from build123d import *

# Parameters (mm, degrees)
F0_W     = 132.985286
F0_H     = 132.985286
F1_DEPTH = 25.4


with BuildPart() as f1:
    # F0 (on Top) → F1 (new body)
    with BuildSketch(Plane.XY):
        Polygon((84.181237, -55.154049), (84.181237, 6.35), (-139.335286, 6.35), (-139.335286, -217.166522), (-77.831237, -217.166522), (-77.831237, -278.670572), (145.685286, -278.670572), (145.685286, -55.154049), align=None)
        Polygon((0, -272.320572), (-71.481237, -272.320572), (-71.481237, -210.816522), (-132.985286, -210.816522), (-132.985286, -139.335286), (0, -139.335286), align=None, mode=Mode.SUBTRACT)
        with Locations((72.842643, -205.827929)):
            Rectangle(F0_W, F0_H, mode=Mode.SUBTRACT)
        with Locations((-66.492643, -66.492643)):
            Rectangle(F0_W, F0_H, mode=Mode.SUBTRACT)
        Polygon((6.35, -132.985286), (6.35, 0), (77.831237, 0), (77.831237, -61.504049), (139.335286, -61.504049), (139.335286, -132.985286), align=None, mode=Mode.SUBTRACT)
    extrude(amount=F1_DEPTH)


solid = f1.part
Could you check a few things on this model? Use its own coordinates, in mm. A direction names the side the tool comes from. Round coordinates to 2 decimals unless told otherwise and drop trailing zeros. Write each loop counter-clockwise with the first axis right and the second up, starting at its lowest first coordinate (ties: lowest second). Pieces come first, ordered by that corner, then holes. Notation, with made-up numbers: (73.5, 88) -> (105.5, 88) arc R31 ccw to (105.5, 113) -> close; hole circle Ø11 at (-24, 66). An arc over 180 degrees is marked (long way). Use a Markdown table: item, result.
1. We'd pull the mould along Y, two halves only. Please class faces 1 (the face through (115, -55.154, 13)), 2 (the face through (-132.985, -67, 13)), 3 (the face through (3, -135, 25.4)): +Y half, -Y half, draft (parallel to the pull), parting line (faces both ways), or undercut.
Answer key:
| item | result |
|---|---|
| face 1 | +Y half |
| face 2 | undercut |
| face 3 | draft |
2. For pin 1 Ø7.5 at (x, z) = (-122, 14) entering from -Y; pin 2 Ø7.5 at (x, z) = (93, 10.5) entering from +Y, each with a flat end and sliding along its axis, tell me the tip position at first contact or that it passes through.
Answer key:
| item | result |
|---|---|
| pin 1 | stops at y = -217.17 |
| pin 2 | stops at y = -55.15 |
3. Please list where these lines run through material, in increasing order: probe 1 along Y at (x, z) = (16, 16.75); probe 2 along Y at (x, z) = (84.5, 8); probe 3 along X at (y, z) = (-193.5, 4.75).
Answer key:
| item | result |
|---|---|
| probe 1 | y = -278.67 to -272.32, -139.34 to -132.99, 0 to 6.35 |
| probe 2 | y = -278.67 to -272.32, -139.34 to -132.99, -61.5 to -55.15 |
| probe 3 | x = -139.34 to -132.99, 0 to 6.35, 139.34 to 145.69 |
4. If we section it at C-C (z = 16.75): List the corners of the cut face in (x, y) for me.
Answer key:
| item | result |
|---|---|
| outline | (-139.34, -217.17) -> (-77.83, -217.17) -> (-77.83, -278.67) -> (145.69, -278.67) -> (145.69, -55.15) -> (84.18, -55.15) -> (84.18, 6.35) -> (-139.34, 6.35) -> close; hole (-132.99, -210.82) -> (-71.48, -210.82) -> (-71.48, -272.32) -> (0, -272.32) -> (0, -139.34) -> (-132.99, -139.34) -> close; hole (-132.99, -132.99) -> (0, -132.99) -> (0, 0) -> (-132.99, 0) -> close; hole (6.35, -272.32) -> (139.34, -272.32) -> (139.34, -139.34) -> (6.35, -139.34) -> close; hole (6.35, -132.99) -> (139.34, -132.99) -> (139.34, -61.5) -> (77.83, -61.5) -> (77.83, 0) -> (6.35, 0) -> close |
5. If we section it at B-B (x = -54.5): List the corners of the cut face in (y, z) for me.
Answer key:
| item | result |
|---|---|
| outline | (-278.67, 0) -> (-272.32, 0) -> (-272.32, 25.4) -> (-278.67, 25.4) -> close; (-139.34, 0) -> (-132.99, 0) -> (-132.99, 25.4) -> (-139.34, 25.4) -> close; (0, 0) -> (6.35, 0) -> (6.35, 25.4) -> (0, 25.4) -> close |
6. If we section it at A-A (y = -89): List the corners of the cut face in (x, z) for me.
Answer key:
| item | result |
|---|---|
| outline | (-139.34, 0) -> (-132.99, 0) -> (-132.99, 25.4) -> (-139.34, 25.4) -> close; (0, 0) -> (6.35, 0) -> (6.35, 25.4) -> (0, 25.4) -> close; (139.34, 0) -> (145.69, 0) -> (145.69, 25.4) -> (139.34, 25.4) -> close |
7. Which directions (+Z, -Z, +X, -X, +Y, -Y) give clear straight access to the entire face, cutting with the end or side of a thin tool? Please do faces 4 (the face through (0, -205, 13)), 5 (the face through (-109, -217.167, 13)), 6 (the face through (-26, 6.35, 13)).
Answer key:
| item | result |
|---|---|
| face 4 | +Z, -Z |
| face 5 | +Z, -Z, -X, -Y |
| face 6 | +Z, -Z, +X, -X, +Y |
